Source: CAD feature listing. Evaluate the final solid. Frame: model axes, mm. A direction names the side the tool comes from. Round coordinates to 2 decimals unless told otherwise and drop trailing zeros. Order: outer loops, then holes, each group sorted by start corner. A loop starts at its lowest first (then second) coordinate and runs counter-clockwise, first axis right, second up. Notation, with made-up numbers: M 70.25,-3 L 106.25,-3 A14 cw 106.25,6 Z; hole C 89.5,77 d1. An arc over 180 degrees is marked long. Answer as CSV lines item,"result". Start each with the question number.
Item 1: Section query A-A on z = 0. Return the cut outline in (x, y), plus the area to 3 significant figures.
Item 2: Section query C-C on y = 103.5. Return the cut outline in (x, z), plus the area to 3 significant figures.
Item 3: Section query D-D on x = -6. Return the cut outline in (y, z).
Item 4: Pull-direction query (X, two-part tool) for faces 1 (the face through (4.5, 0, 7)), 2 (the face through (10, 0, -5.5)), 3 (the face through (-8.5, 0, -7)), 4 (the face through (-4.5, 0, 7)); classes: +X half, -X half, draft (parallel to the pull), parting line (faces both ways), or undercut.
Item 5: Section query B-B on x = 6.5. Return the cut outline in (y, z).
Item 6: Set-up query: faces 5 (the face through (8.5, 0, -7)), 6 (the face through (-10, 0, 5.5)), 7 (the face through (-4.5, 0, -7)), 8 (the face through (10, 0, 5.5)). Return all of +Z, -Z, +X, -X, +Y, -Y with unobstructed straight access to the full face (end or side cutting, diameter ignored); none if empty.
Item 7: First-contact query: P1, Ø1, axis at x = 10, y = 0.5, coming from the -Z side; P2, Ø0.6, axis at x = 1.5, y = 0, coming from the +Z side; P3, Ø8.5, axis at x = 4, z = -1, coming from the +Y side; P4, Ø1.6, axis at y = 0, z = -6.5, coming from the +X side. Flat tips, straight axial feed; report the tip coordinate or a pass-through.
Item 8: Line query: line 1 (Y direction, x = 8, z = 1.5); line 2 (Z direction, x = 8.25, y = 70); line 3 (Z direction, x = 7.25, y = 97.5). Output: solid intervals per line, ascending. Write a range as [from, to].
from build123d import *

# Parameters (mm, degrees)
SKETCH1_W           = 23
SKETCH1_H           = 11
BOSS_EXTRUDE1_DEPTH = 1
SKETCH3_W           = 4
SKETCH3_H           = 3
BOSS_EXTRUDE3_DEPTH = 1
SKETCH2_R           = 2
BOSS_EXTRUDE2_DEPTH = 115


with BuildPart() as part:
    # Sketch1 → Boss-Extrude1 (new, symmetric)
    with BuildSketch(Plane(origin=(0, 0, 0), x_dir=(1, 0, 0), z_dir=(0, 1, 0))):
        Rectangle(SKETCH1_W, SKETCH1_H)
    extrude(amount=BOSS_EXTRUDE1_DEPTH, both=True)

    # Sketch3 → Boss-Extrude3 (add, symmetric)
    with BuildSketch(Plane(origin=(0, 0, 0), x_dir=(1, 0, 0), z_dir=(0, 1, 0))):
        with Locations((6.5, 7)):
            Rectangle(SKETCH3_W, SKETCH3_H)
        with Locations((6.5, -7)):
            Rectangle(SKETCH3_W, SKETCH3_H)
        with Locations((-6.5, -7)):
            Rectangle(SKETCH3_W, SKETCH3_H)
        with Locations((-6.5, 7)):
            Rectangle(SKETCH3_W, SKETCH3_H)
    extrude(amount=BOSS_EXTRUDE3_DEPTH, both=True)

    # Sketch2 → Boss-Extrude2 (add)
    with BuildSketch(Plane(origin=(0, 1, 0), x_dir=(1, 0, 0), z_dir=(0, 1, 0))):
        with Locations(Location((6.5, 0, 0), (0, 0, 270))):
            Circle(SKETCH2_R)
    extrude(amount=BOSS_EXTRUDE2_DEPTH)


solid = part.part
Results:
1,outline,"M -11.5,-1 L 11.5,-1 L 11.5,1 L 8.5,1 L 8.5,116 L 4.5,116 L 4.5,1 L -11.5,1 Z"
1,area,"506 mm^2"
2,outline,"C 6.5,0 d4"
2,area,"12.6 mm^2"
3,outline,"M -1,-8.5 L 1,-8.5 L 1,8.5 L -1,8.5 Z"
4,face 1,"undercut"
4,face 2,"draft"
4,face 3,"-X half"
4,face 4,"undercut"
5,outline,"M -1,-8.5 L 1,-8.5 L 1,-2 L 116,-2 L 116,2 L 1,2 L 1,8.5 L -1,8.5 Z"
6,face 5,"-Z, +X, +Y, -Y"
6,face 6,"+Z, -X, +Y, -Y"
6,face 7,"-Z, +Y, -Y"
6,face 8,"+Z, +X, +Y, -Y"
7,P1,"z = -5.5"
7,P2,"z = 5.5"
7,P3,"y = 116"
7,P4,"x = 8.5"
8,line 1,"[-1, 1]"
8,line 2,"[-0.97, 0.97]"
8,line 3,"[-1.85, 1.85]"
